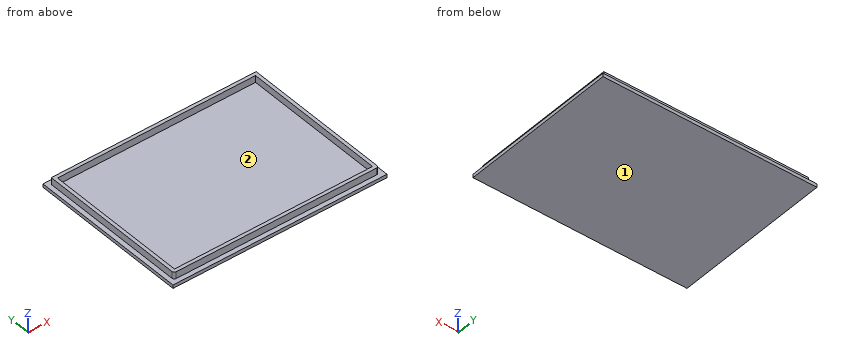
from build123d import *

# Parameters (mm, degrees)
BOX001_W     = 90
BOX001_H     = 66
BOX001_DEPTH = 4.5
THICKNESS_T  = -1.5
FILLET001_R  = 1.5
BOX_W        = 94
BOX_H        = 70
BOX_DEPTH    = 1.5
FILLET_R     = 1
FILLET002_R  = 1


with BuildPart() as thickness:
    # Box001 → Box001 (new body)
    with BuildSketch(Plane(origin=(2, 2, 0), x_dir=(1, 0, 0), z_dir=(0, 0, 1))):
        with Locations((45, 33)):
            Rectangle(BOX001_W, BOX001_H)
    extrude(amount=BOX001_DEPTH)

    # Thickness
    thickness_openings = [thickness.faces().sort_by_distance(p)[0] for p in [
        (47, 35, 4.5),
    ]]
    offset(amount=THICKNESS_T, openings=thickness_openings)


with BuildPart() as fillet001:
    # Fillet001 base: copy of Thickness
    add(thickness.part)

    # Fillet001
    fillet001_edges = [fillet001.edges().sort_by_distance(p)[0] for p in [
        (92, 2, 2.25),
        (2, 2, 2.25),
    ]]
    fillet(fillet001_edges, radius=FILLET001_R)


with BuildPart() as obj1:
    # Box → Box (new body)
    with BuildSketch(Plane.XY):
        with Locations((47, 35)):
            Rectangle(BOX_W, BOX_H)
    extrude(amount=BOX_DEPTH)


with BuildPart() as fusion001:
    # Fillet base: copy of Thickness
    add(thickness.part)

    # Fillet
    fillet_edges = [fusion001.edges().sort_by_distance(p)[0] for p in [
        (92, 2, 2.25),
        (2, 2, 2.25),
    ]]
    fillet(fillet_edges, radius=FILLET_R)

    # Fillet002
    fillet002_edges = [fusion001.edges().sort_by_distance(p)[0] for p in [
        (92, 68, 2.25),
        (2, 68, 2.25),
    ]]
    fillet(fillet002_edges, radius=FILLET002_R)

    # Fusion: union Fillet001, obj1
    add(fillet001.part)
    add(obj1.part)


solid = fusion001.part
The listing builds one solid part. Answer for the finished solid, in the listing's coordinates (mm). Face numbers are marked on the shaded views. Coordinates: 2 decimals unless noted, no trailing zeros. Write each loop counter-clockwise with the first axis right and the second up, starting at its lowest first coordinate (ties: lowest second). Pieces come first, ordered by that corner, then holes. Notation, with made-up numbers: (-29.5, -5) - (10.5, -5) arc R30 cw to (10.5, 22) - close; hole circle Ø10 at (12.5, 21). An arc over 180 degrees is marked (long way). Answer as CSV lines item,"result".
1. Straight lines are drawn through the part: line 1 (X direction, y = 57.5, z = 3.8); line 2 (Y direction, x = 22, z = 1.95); line 3 (Z direction, x = 32.5, y = 31). For each, find the intervals that lie inside material, in ascending order. Write a range as [from, to].
Computed values:
line 1,"x = [2, 3.5], [90.5, 92]"
line 2,"y = [2, 3.5], [66.5, 68]"
line 3,"z = [0, 1.5]"
2. Find section A-A (z = 2.35). Give the vertices of the cut face in (x, y), plus the area to 3 significant figures.
Computed values:
outline,"(2, 3) arc R1 ccw to (3, 2) - (91, 2) arc R1 ccw to (92, 3) - (92, 68) - (2, 68) - close; hole (3.5, 3.5) - (90.5, 3.5) - (90.5, 66.5) - (3.5, 66.5) - close"
area,"459 mm²"
3. Given P1, Ø1.5, axis at y = 40, z = 3, coming from the -X side; P2, Ø0.9, axis at x = 65, z = 3.5, coming from the -Y side; P3, Ø0.9, axis at y = 49, z = 2.5, coming from the +X side, each flat-ended and moving along its own axis, determine where each tip first touches the part or whether it passes through.
Computed values:
P1,"stops at x = 2"
P2,"stops at y = 2"
P3,"stops at x = 92"
4. Find section C-C (x = 30). Give the vertices of the cut face in (y, z).
Computed values:
outline,"(0, 0) - (70, 0) - (70, 1.5) - (68, 1.5) - (68, 4.5) - (66.5, 4.5) - (66.5, 1.5) - (3.5, 1.5) - (3.5, 4.5) - (2, 4.5) - (2, 1.5) - (0, 1.5) - close"
5. Find section B-B (y = 5). Give the vertices of the cut face in (x, z), plus the area to 3 significant figures.
Computed values:
outline,"(0, 0) - (94, 0) - (94, 1.5) - (92, 1.5) - (92, 4.5) - (90.5, 4.5) - (90.5, 1.5) - (3.5, 1.5) - (3.5, 4.5) - (2, 4.5) - (2, 1.5) - (0, 1.5) - close"
area,"150 mm²"
6. Determine the mould class of the marked faces 1 and 2 for opening direction Y: +Y half, -Y half, draft (parallel to the pull), parting line (faces both ways), or undercut.
Computed values:
face 1,"draft"
face 2,"undercut"
